Geometry: see drawing. Coordinates: mm, zero at the bounding-box minimum. Give positions to 0.01 mm unless a question says otherwise; leave off trailing zeros. Order: outer loops, then holes, each group sorted by start corner. A loop starts at its lowest first (then second) coordinate and runs counter-clockwise, first axis right, second up. Notation, with made-up numbers: (47, -5) - (63, -5) arc R15 ccw to (63, 6) - close; hole circle Ø11 at (49, -31). An arc over 180 degrees is marked (long way). Write item = value, one per line. Start each with the question number.
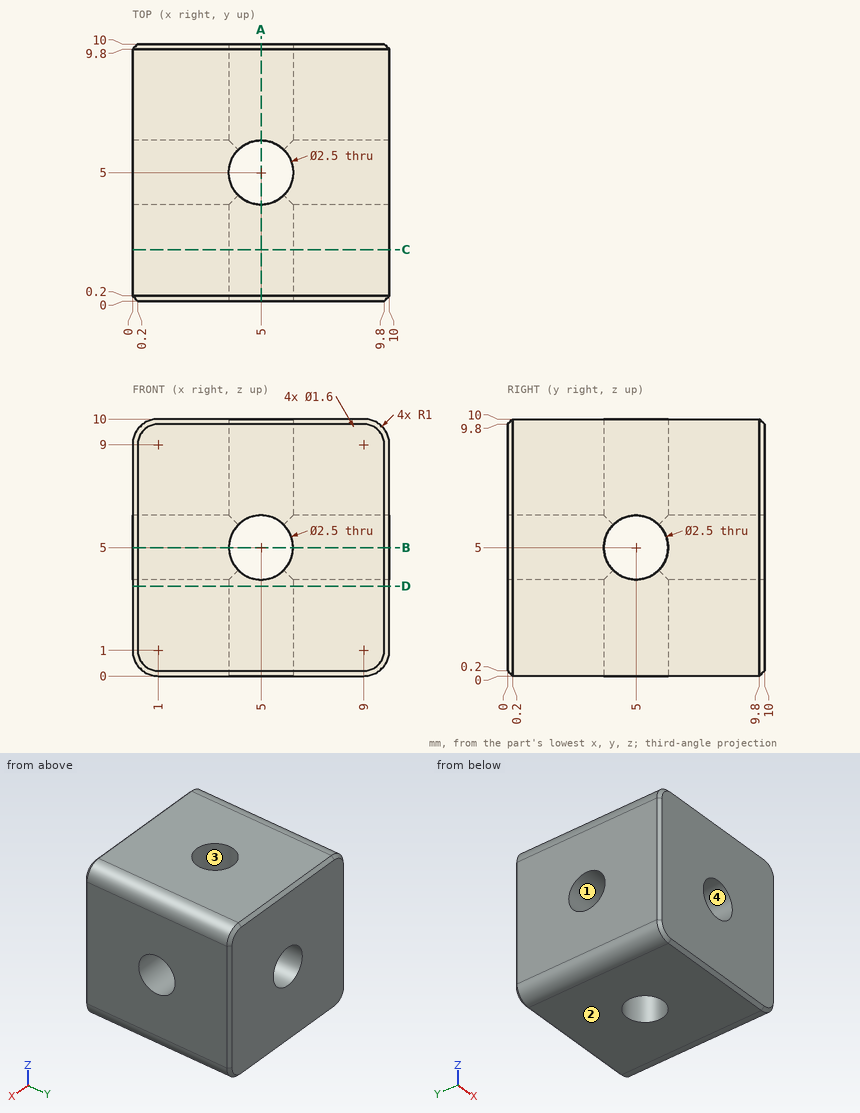
Q1. Section A-A, the plane x = 5. Return the cut outline in (y, z).
Q2. Pull-direction query (Z, two-part tool) for the marked faces 1, 2, 3 and 4; classes: +Z half, -Z half, draft (parallel to the pull), parting line (faces both ways), or undercut.
Q3. Section C-C, the plane y = 2. Return the cut outline in (x, z).
Q4. Section D-D, the plane z = 3.5. Return the cut outline in (x, y), then the cut area to 3 significant figures.
Q5. Material intervals for line 1 along Y through (x, z) = (3.15, 5); line 2 along Y through (x, z) = (6, 0.5), sorted ascending. Write a range as from..to.
The answers:
q1.outline = (0, 0.2) - (0.2, 0) - (3.75, 0) - (3.75, 3.75) - (0, 3.75) - close; (0, 6.25) - (3.75, 6.25) - (3.75, 10) - (0.2, 10) - (0, 9.8) - close; (6.25, 0) - (9.8, 0) - (10, 0.2) - (10, 3.75) - (6.25, 3.75) - close; (6.25, 6.25) - (10, 6.25) - (10, 9.8) - (9.8, 10) - (6.25, 10) - close
q2.face_1 = undercut
q2.face_2 = -Z half
q2.face_3 = draft
q2.face_4 = undercut
q3.outline = (0, 1) arc R1 ccw to (1, 0) - (9, 0) arc R1 ccw to (10, 1) - (10, 9) arc R1 ccw to (9, 10) - (1, 10) arc R1 ccw to (0, 9) - close; hole circle Ø2.5 at (5, 5)
q4.outline = (0, 0.2) - (0.2, 0) - (9.8, 0) - (10, 0.2) - (10, 9.8) - (9.8, 10) - (0.2, 10) - (0, 9.8) - close; hole circle Ø2.5 at (5, 5)
q4.area = 95.0 mm²
q5.line_1 = 0..3.75, 6.25..10
q5.line_2 = 0..4.25, 5.75..10
